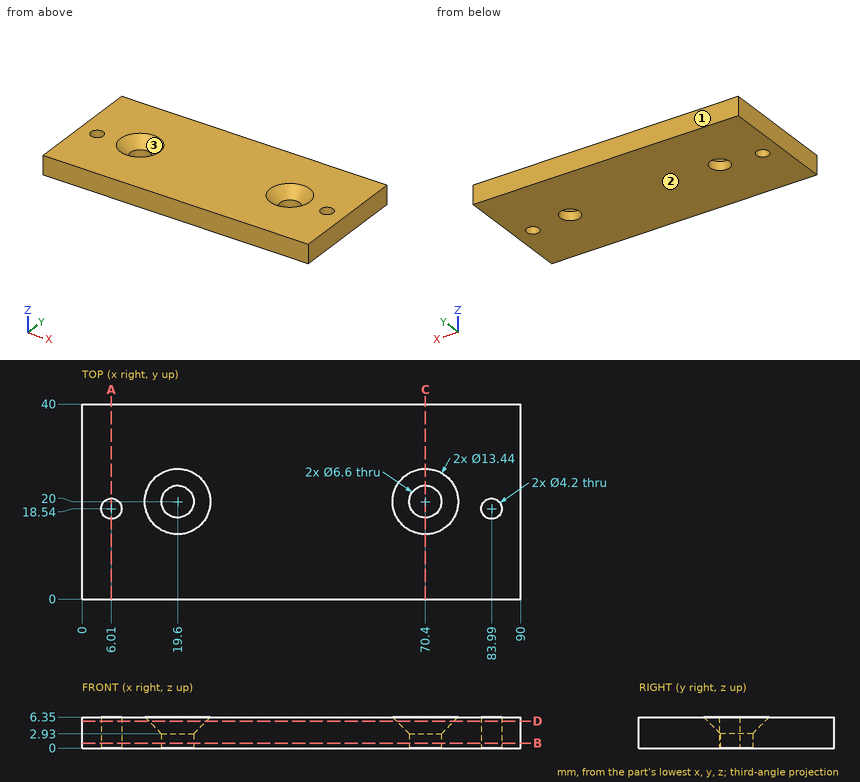
Check sheet for the drawn part. Datum: minimum x, y, z corner. Units: mm. Round coordinates to 2 decimals unless told otherwise and drop trailing zeros. Write each loop counter-clockwise with the first axis right and the second up, starting at its lowest first coordinate (ties: lowest second). Pieces come first, ordered by that corner, then holes. Notation, with made-up numbers: (77.5, 21.5) -> (91.5, 21.5) arc R20 cw to (91.5, 30.5) -> close; hole circle Ø10 at (75.5, 13.5). An arc over 180 degrees is marked (long way). One line per item, written item: value. Start each with the question number.
(1) Scan lines: line 1 (Y direction, x = 19.6, z = 1.05); line 2 (X direction, y = 20, z = 2); line 3 (X direction, y = 24, z = 5.25). Record each from-to range of solid material in increasing order. Write a range as [from, to].
(2) Cross-section at C-C, the plane x = 70.4. Record the cut outline in (y, z).
(3) Draft check along Y on the marked faces 1, 2 and 3. Enter one of: +Y half, -Y half, draft (parallel to the pull), parting line (faces both ways), or undercut.
(4) Go/stop test with flat-tipped pins: pin 1 Ø4 at (x, y) = (83.99, 18.54) entering from -Z; pin 2 Ø7.5 at (x, y) = (19.6, 20) entering from +Z. Record where each tip stops, or that it passes through.
(5) Cross-section at D-D, the plane z = 5.5. Record the cut outline in (x, y).
(6) Cross-section at B-B, the plane z = 1. Record the cut outline in (x, y), and give its area (3 significant figures).
(7) Cross-section at A-A, the plane x = 6.01. Record the cut outline in (y, z), and give its area (3 significant figures).
Answer:
1. line 1: [0, 16.7], [23.3, 40]
1. line 2: [0, 4.5], [7.52, 16.3], [22.9, 67.1], [73.7, 82.48], [85.5, 90]
1. line 3: [0, 15.65], [23.55, 66.45], [74.35, 90]
2. outline: (0, 0) -> (16.7, 0) -> (16.7, 2.93) -> (13.28, 6.35) -> (0, 6.35) -> close; (23.3, 0) -> (40, 0) -> (40, 6.35) -> (26.72, 6.35) -> (23.3, 2.93) -> close
3. face 1: +Y half
3. face 2: draft
3. face 3: undercut
4. pin 1: through
4. pin 2: z = 3.38
5. outline: (0, 0) -> (90, 0) -> (90, 40) -> (0, 40) -> close; hole circle Ø4.2 at (6.01, 18.54); hole circle Ø11.74 at (19.6, 20); hole circle Ø11.74 at (70.4, 20); hole circle Ø4.2 at (83.99, 18.54)
6. outline: (0, 0) -> (90, 0) -> (90, 40) -> (0, 40) -> close; hole circle Ø4.2 at (6.01, 18.54); hole circle Ø6.6 at (19.6, 20); hole circle Ø6.6 at (70.4, 20); hole circle Ø4.2 at (83.99, 18.54)
6. area: 3,500 mm²
7. outline: (0, 0) -> (16.44, 0) -> (16.44, 6.35) -> (0, 6.35) -> close; (20.64, 0) -> (40, 0) -> (40, 6.35) -> (20.64, 6.35) -> close
7. area: 227 mm²
